from build123d import *

# Parameters (mm, degrees)
F1_DEPTH = 25
F3_R     = 2
F4_DEPTH = 10
F2_R     = 2
F5_DEPTH = 50
F6_R     = 5
F7_R     = 2
F8_DEPTH = 3


with BuildPart() as f1:
    # F0 (on Top) → F1 (new body)
    with BuildSketch(Plane.XY):
        with BuildLine():
            ThreePointArc((10, 12.4899959968), (14.4222051019, 6.9282032303), (16, 0))
            ThreePointArc((16, 0), (-6.9282032303, -14.4222051019), (-10, 12.4899959968))
            Line((-10, 12.4899959968), (-10, 21.8174242293))
            ThreePointArc((-10, 21.8174242293), (-21.7833717136, 10.0739623181), (-23.1002589039, -6.5098416703))
            ThreePointArc((-23.1002589039, -6.5098416703), (-19.1230344611, -14.5020534064), (-12.5, -20.4878012485))
            Line((-12.5, -20.4878012485), (-12.5, -19.125))
            Line((-12.5, -19.125), (12.5, -19.125))
            Line((12.5, -19.125), (12.5, -20.4878012485))
            ThreePointArc((12.5, -20.4878012485), (19.1230344611, -14.5020534064), (23.1002589039, -6.5098416703))
            ThreePointArc((23.1002589039, -6.5098416703), (23.7740006488, -3.2858626193), (24, 0))
            ThreePointArc((24, 0), (20.1990098767, 12.9614813968), (10, 21.8174242293))
            Line((10, 21.8174242293), (10, 12.4899959968))
        make_face()
        with BuildLine():
            Line((-10, 21.8174242293), (-10, 12.4899959968))
            ThreePointArc((-10, 12.4899959968), (-6.4658560997, 14.635323874), (-2.5, 15.8034806293))
            Line((-2.5, 15.8034806293), (-2.5, 23.8694365246))
            ThreePointArc((-2.5, 23.8694365246), (-6.3336552334, 23.1491859767), (-10, 21.8174242293))
        make_face()
        with BuildLine():
            Line((-10, 38.3634492755), (-10, 21.8174242293))
            ThreePointArc((-10, 21.8174242293), (-6.3336552334, 23.1491859767), (-2.5, 23.8694365246))
            Line((-2.5, 23.8694365246), (-2.5, 38.3634492755))
            Line((-2.5, 38.3634492755), (-10, 38.3634492755))
        make_face()
        with BuildLine():
            ThreePointArc((2.5, 15.8034806293), (6.4658560997, 14.635323874), (10, 12.4899959968))
            Line((10, 12.4899959968), (10, 21.8174242293))
            ThreePointArc((10, 21.8174242293), (6.3336552334, 23.1491859767), (2.5, 23.8694365246))
            Line((2.5, 23.8694365246), (2.5, 15.8034806293))
        make_face()
        with BuildLine():
            ThreePointArc((2.5, 23.8694365246), (6.3336552334, 23.1491859767), (10, 21.8174242293))
            Line((10, 21.8174242293), (10, 38.3634492755))
            Line((10, 38.3634492755), (2.5, 38.3634492755))
            Line((2.5, 38.3634492755), (2.5, 23.8694365246))
        make_face()
        with BuildLine():
            Line((-12.5, -19.125), (-12.5, -20.4878012485))
            ThreePointArc((-12.5, -20.4878012485), (-6.492024724, -23.1052724499), (0, -24))
            ThreePointArc((0, -24), (6.492024724, -23.1052724499), (12.5, -20.4878012485))
            Line((12.5, -20.4878012485), (12.5, -19.125))
            Line((12.5, -19.125), (-12.5, -19.125))
        make_face()
        with BuildLine():
            ThreePointArc((-12.5, -20.4878012485), (-19.1230344611, -14.5020534064), (-23.1002589039, -6.5098416703))
            Line((-23.1002589039, -6.5098416703), (-12.5, -44.125))
            Line((-12.5, -44.125), (-12.5, -20.4878012485))
        make_face()
        with BuildLine():
            ThreePointArc((0, -24), (-6.492024724, -23.1052724499), (-12.5, -20.4878012485))
            Line((-12.5, -20.4878012485), (-12.5, -44.125))
            Line((-12.5, -44.125), (12.5, -44.125))
            Line((12.5, -44.125), (12.5, -20.4878012485))
            ThreePointArc((12.5, -20.4878012485), (6.492024724, -23.1052724499), (0, -24))
        make_face()
        Polygon((-7.625, -24), (0, -24), (7.625, -24), (7.625, -39.25), (-7.625, -39.25), align=None, mode=Mode.SUBTRACT)
        with BuildLine():
            Line((12.5, -44.125), (23.1002589039, -6.5098416703))
            ThreePointArc((23.1002589039, -6.5098416703), (19.1230344611, -14.5020534064), (12.5, -20.4878012485))
            Line((12.5, -20.4878012485), (12.5, -44.125))
        make_face()
    extrude(amount=F1_DEPTH)

    # F3 (on face) → F4 (cut)
    with BuildSketch(Plane.XZ.offset(44.125)):
        with Locations((0, 7)):
            Circle(F3_R)
        with Locations((0, 18)):
            Circle(F3_R)
    extrude(amount=-F4_DEPTH, mode=Mode.SUBTRACT)

    # F2 (on face) → F5 (cut)
    with BuildSketch(Plane.YZ.offset(10)):
        with Locations((30.0904367524, 18)):
            Circle(F2_R)
        with Locations((30.0904367524, 7)):
            Circle(F2_R)
    extrude(amount=-F5_DEPTH, mode=Mode.SUBTRACT)

    # F6
    f6_edges = [f1.edges().sort_by_distance(p)[0] for p in [
        (12.5, -44.125, 12.5),
        (-12.5, -44.125, 12.5),
        (10, 21.817424, 12.5),
        (-10, 21.817424, 12.5),
        (-2.5, 15.803481, 12.5),
        (2.5, 15.803481, 12.5),
    ]]
    fillet(f6_edges, radius=F6_R)

    # F7
    f7_edges = [f1.edges().sort_by_distance(p)[0] for p in [
        (10, 38.363449, 12.5),
        (-10, 38.363449, 12.5),
        (-2.5, 38.363449, 12.5),
        (2.5, 38.363449, 12.5),
    ]]
    fillet(f7_edges, radius=F7_R)

    # F2 (on face) → F8 (cut)
    with BuildSketch(Plane.YZ.offset(10)):
        Polygon((33.4679358271, 18), (31.7791862898, 20.925), (28.401687215, 20.925), (26.7129376776, 18), (28.401687215, 15.075), (31.7791862898, 15.075), align=None)
        with Locations((30.0904367524, 18)):
            Circle(F2_R, mode=Mode.SUBTRACT)
        Polygon((33.4679337645, 7.0037327168), (31.7759526309, 9.9268645721), (28.3984556188, 9.9231318553), (26.7129397403, 6.9962672832), (28.4049208739, 4.0731354279), (31.782417886, 4.0768681447), align=None)
        with Locations((30.0904367524, 7)):
            Circle(F2_R, mode=Mode.SUBTRACT)
    extrude(amount=-F8_DEPTH, mode=Mode.SUBTRACT)


solid = f1.part
Input: part model. Units: mm. Frame: model coordinates. A direction names the side the tool comes from. Round coordinates to 2 decimals unless told otherwise and drop trailing zeros. Order: outer loops, then holes, each group sorted by start corner. A loop starts at its lowest first (then second) coordinate and runs counter-clockwise, first axis right, second up.
1. Cut plane D-D, the plane x = -21. Output: boundary loops of the cut face in (y, z), then the cut area to 3 significant figures.
The answers:
outline: (-13.96, 0) - (11.62, 0) - (11.62, 25) - (-13.96, 25) - close
area: 640 mm2
2. Mould query, pull axis Y, two halves, no side actions, for faces 1 (the face through (10, 31, 12)), 2 (the face through (10.663, 22.332, 12.675)), 3 (the face through (3.405, 16.746, 12.675)). Classes: released by +Y, released by -Y, zero draft, split by the parting line, or undercut.
The answers:
face 1: zero draft
face 2: released by +Y
face 3: undercut
3. Cut plane B-B, the plane x = 0. Output: boundary loops of the cut face in (y, z) (3 decimals).
The answers:
outline: (-44.125, 0) - (-39.25, 0) - (-39.25, 5) - (-44.125, 5) - close; (-44.125, 9) - (-39.25, 9) - (-39.25, 16) - (-44.125, 16) - close; (-44.125, 20) - (-39.25, 20) - (-39.25, 25) - (-44.125, 25) - close; (-24, 0) - (-16, 0) - (-16, 25) - (-24, 25) - close
4. Set-up query: faces 4 (the face through (0, -39.25, 12)), 5 (the face through (-2.5, 28, 12)), 6 (the face through (6, 38.363, 12)), 7 (the face through (8.5, 32.6, 5.5)). Return all of +Z, -Z, +X, -X, +Y, -Y with unobstructed straight access to the full face (end or side cutting, diameter ignored); none if empty.
The answers:
face 4: +Z, -Z
face 5: +Z, -Z, +Y
face 6: +Z, -Z, +X, -X, +Y
face 7: +X
5. Pin query (flat end, axial travel): P1, Ø9, axis at y = 29, z = 11.5, coming from the +X side; P2, Ø6, axis at y = 5, z = 13.5, coming from the -X side; P3, Ø5, axis at x = 0, z = 18, coming from the -Y side (3 decimals); P4, Ø1.5, axis at y = -19.5, z = 16.5, coming from the +X side. Return the tip coordinate at first contact, or that it passes through.
The answers:
P1: stops at x = 10.01
P2: stops at x = -23.92
P3: stops at y = -44.125
P4: stops at x = 19.65
6. Cut plane A-A, the plane z = 11. Output: boundary loops of the cut face in (x, y) (3 decimals).
The answers:
outline: (-23.1, -6.51) - (-13.527, -40.481) arc R5 ccw to (-8.714, -44.125) - (8.714, -44.125) arc R5 ccw to (13.527, -40.481) - (23.1, -6.51) arc R24 ccw to (12.414, 20.54) arc R5 cw to (10, 24.819) - (10, 36.363) arc R2 ccw to (8, 38.363) - (4.5, 38.363) arc R2 ccw to (2.5, 36.363) - (2.5, 19.615) arc R5 ccw to (5.714, 14.945) arc R16 cw (long way) to (-5.714, 14.945) arc R5 ccw to (-2.5, 19.615) - (-2.5, 36.363) arc R2 ccw to (-4.5, 38.363) - (-8, 38.363) arc R2 ccw to (-10, 36.363) - (-10, 24.819) arc R5 cw to (-12.414, 20.54) arc R24 ccw to start; hole (-7.625, -39.25) - (7.625, -39.25) - (7.625, -24) - (-7.625, -24) - close
7. Material intervals for line 1 (Y direction, x = 0, z = 9.75) (3 decimals); line 2 (X direction, y = 0, z = 18); line 3 (Y direction, x = -6, z = 4.75) (3 decimals), sorted ascending.
The answers:
line 1: y = -44.125 to -39.25, -24 to -16
line 2: x = -24 to -16, 16 to 24
line 3: y = -44.125 to -39.25, -24 to -14.832, 14.832 to 38.363
8. Cut plane C-C, the plane y = -13. Output: boundary loops of the cut face in (x, z), then the cut area to 3 significant figures.
The answers:
outline: (-21.27, 0) - (-9.33, 0) - (-9.33, 25) - (-21.27, 25) - close; (9.33, 0) - (21.27, 0) - (21.27, 25) - (9.33, 25) - close
area: 597 mm2
